Study the drawing (mm; zero at the part's minimum x, y, z) and answer. Coordinates: 2 decimals unless noted, no trailing zeros. Loops run counter-clockwise (first coordinate to the right, second up) from the corner with the lowest first, then second, coordinate; pieces in that order, holes last. Notation, with made-up numbers: (-18.5, 25.5) -> (23.5, 25.5) arc R15 ccw to (23.5, 39.5) -> close; hole circle Ø2 at (38.25, -18). An arc over 180 degrees is marked (long way). One line per question, with ' | ' between items.
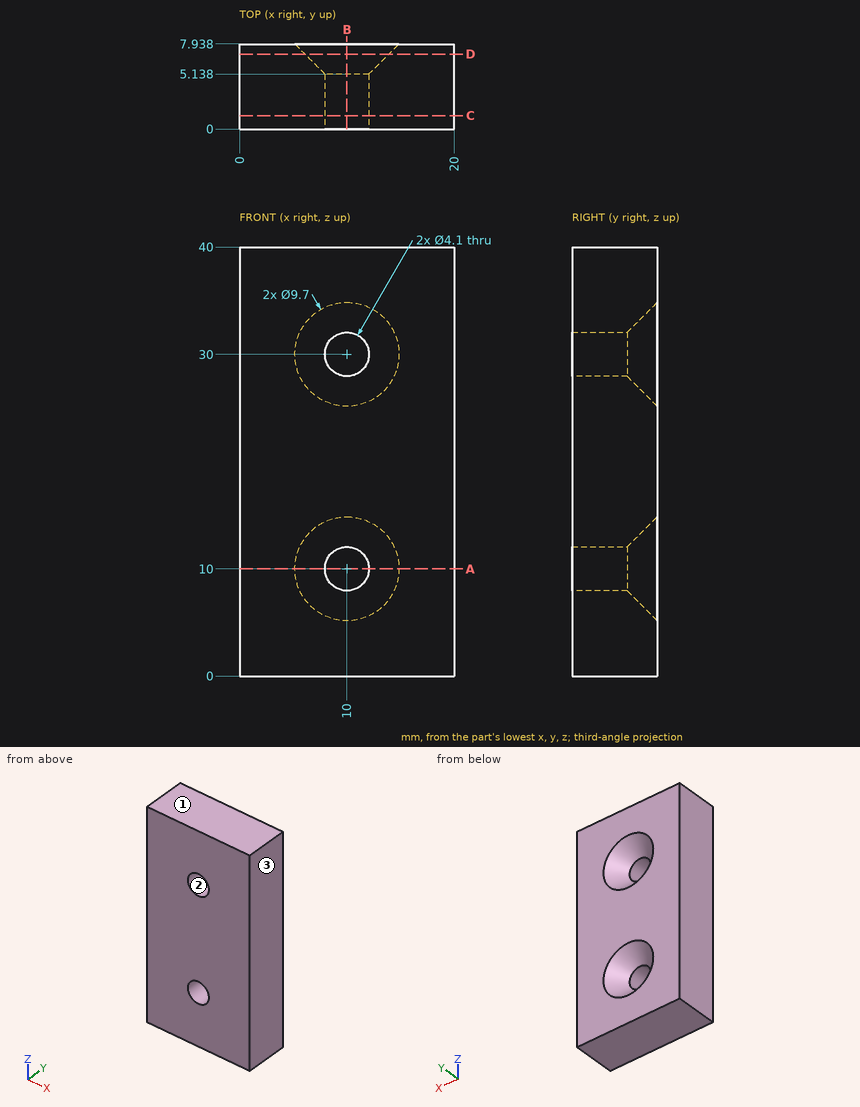
1) Find section A-A (z = 10). Write down the section's boundary in (x, y), plus the area to 3 significant figures.
Check values:
outline: (0, 0) -> (7.95, 0) -> (7.95, 5.14) -> (5.15, 7.94) -> (0, 7.94) -> close; (12.05, 0) -> (20, 0) -> (20, 7.94) -> (14.85, 7.94) -> (12.05, 5.14) -> close | area: 118 mm^2
2) Find the intervals of material crossed by line 1 along Z through (x, y) = (10, 1.55); line 2 along X through (y, z) = (2.65, 10); line 3 along Z through (x, y) = (11.25, 2.5) (1 decimal), in increasing order.
Check values:
line 1: z = 0 to 7.95, 12.05 to 27.95, 32.05 to 40 | line 2: x = 0 to 7.95, 12.05 to 20 | line 3: z = 0 to 8.4, 11.6 to 28.4, 31.6 to 40
3) Find section D-D (y = 7). Write down the section's boundary in (x, z) (1 decimal), plus the area to 3 significant figures.
Check values:
outline: (0, 0) -> (20, 0) -> (20, 40) -> (0, 40) -> close; hole circle Ø7.8 at (10, 10); hole circle Ø7.8 at (10, 30) | area: 704 mm^2
4) The mould has two halves that part along Z. Classify the marked faces 1, 2 and 3: released by +Z, released by -Z, zero draft, split by the parting line, or undercut.
Check values:
face 1: released by +Z | face 2: undercut | face 3: zero draft
5) Find section B-B (x = 10). Write down the section's boundary in (y, z), plus the area to 3 significant figures.
Check values:
outline: (0, 0) -> (7.94, 0) -> (7.94, 5.15) -> (5.14, 7.95) -> (0, 7.95) -> close; (0, 12.05) -> (5.14, 12.05) -> (7.94, 14.85) -> (7.94, 25.15) -> (5.14, 27.95) -> (0, 27.95) -> close; (0, 32.05) -> (5.14, 32.05) -> (7.94, 34.85) -> (7.94, 40) -> (0, 40) -> close | area: 237 mm^2
6) Find section C-C (y = 1.25). Write down the section's boundary in (x, z).
Check values:
outline: (0, 0) -> (20, 0) -> (20, 40) -> (0, 40) -> close; hole circle Ø4.1 at (10, 10); hole circle Ø4.1 at (10, 30)
